```python
from build123d import *
from OCP.BRepFilletAPI import BRepFilletAPI_MakeChamfer

# Parameters (mm, degrees)
SKETCH1_W           = 46
SKETCH1_H           = 34
SKETCH1_R           = 4.5
BOSS_EXTRUDE1_DEPTH = 17
SKETCH2_W           = 45.8
SKETCH2_H           = 33.8
BOSS_EXTRUDE2_DEPTH = 2
SKETCH3_W           = 45.8
SKETCH3_H           = 33.8
BOSS_EXTRUDE3_DEPTH = 5
CHAMFER1_SIZE       = 5
CHAMFER1_SIZE2      = 4.346433689
SKETCH5_R           = 4.5
CUT_EXTRUDE1_DEPTH  = 63.032249677
CUT_EXTRUDE2_DEPTH  = 4
CUT_EXTRUDE3_DEPTH  = 4.5
CUT_EXTRUDE4_DEPTH  = 0.2
SKETCH11_W          = 11.4
SKETCH11_H          = 5
BOSS_EXTRUDE4_DEPTH = 4
SKETCH12_W          = 10.4
SKETCH12_H          = 1
CUT_EXTRUDE5_DEPTH  = 0.5
SKETCH13_W          = 10.4
SKETCH13_H          = 3
CUT_EXTRUDE6_DEPTH  = 0.5
SKETCH14_W          = 0.75
SKETCH14_H          = 2
BOSS_EXTRUDE5_DEPTH = 0.5
SKETCH15_W          = 0.75
SKETCH15_H          = 1
BOSS_EXTRUDE6_DEPTH = 1
SKETCH16_W          = 10.4
SKETCH16_H          = 3
BOSS_EXTRUDE7_DEPTH = 1
CUT_EXTRUDE7_DEPTH  = 1
SKETCH19_R          = 1
CUT_EXTRUDE8_DEPTH  = 2
SKETCH20_R          = 1.848835828
CUT_EXTRUDE9_DEPTH  = 2
BOSS_EXTRUDE8_DEPTH = 2
BOSS_EXTRUDE9_DEPTH = 2


with BuildPart() as part:
    # Sketch1 → Boss-Extrude1 (new body)
    with BuildSketch(Plane(origin=(0, 0, 0), x_dir=(1, 0, 0), z_dir=(0, 1, 0))):
        with Locations((23, 17)):
            Rectangle(SKETCH1_W, SKETCH1_H)
        with Locations(Location((23, 17, 0), (0, 0, 270))):
            Circle(SKETCH1_R, mode=Mode.SUBTRACT)
    extrude(amount=BOSS_EXTRUDE1_DEPTH)

    # Sketch2 → Boss-Extrude2 (add)
    with BuildSketch(Plane(origin=(0, 17, 0), x_dir=(1, 0, 0), z_dir=(0, 1, 0))):
        with Locations((23, 17)):
            Rectangle(SKETCH2_W, SKETCH2_H)
    extrude(amount=BOSS_EXTRUDE2_DEPTH)

    # Sketch3 → Boss-Extrude3 (add)
    with BuildSketch(Plane(origin=(0, 19, 0), x_dir=(1, 0, 0), z_dir=(0, 1, 0))):
        with Locations((23, 17)):
            Rectangle(SKETCH3_W, SKETCH3_H)
    extrude(amount=BOSS_EXTRUDE3_DEPTH)

    # Chamfer1: one chamfer whose edges measure the first distance from different faces: ONE call of the kernel's chamfer builder (chamfer() names one face for all edges)
    chamfer1_edges_1 = [part.edges().sort_by_distance(p)[0] for p in [
        (23, 24, -33.9),
    ]]
    chamfer1_side_1 = [part.faces().sort_by_distance(p)[0] for p in [
        (23, 20.5, -33.9),
    ]]
    chamfer1_edges_2 = [part.edges().sort_by_distance(p)[0] for p in [
        (0.1, 24, -17),
    ]]
    chamfer1_side_2 = [part.faces().sort_by_distance(p)[0] for p in [
        (0.1, 20.5, -17),
    ]]
    chamfer1_edges_3 = [part.edges().sort_by_distance(p)[0] for p in [
        (23, 24, -0.1),
    ]]
    chamfer1_side_3 = [part.faces().sort_by_distance(p)[0] for p in [
        (23, 20.5, -0.1),
    ]]
    chamfer1_edges_4 = [part.edges().sort_by_distance(p)[0] for p in [
        (45.9, 24, -17),
    ]]
    chamfer1_side_4 = [part.faces().sort_by_distance(p)[0] for p in [
        (45.9, 20.5, -17),
    ]]
    chamfer1 = BRepFilletAPI_MakeChamfer(part.part.solid().wrapped)
    for e in chamfer1_edges_1:
        chamfer1.Add(CHAMFER1_SIZE, CHAMFER1_SIZE2, e.wrapped, chamfer1_side_1[0].wrapped)  # the first distance lies on this face
    for e in chamfer1_edges_2:
        chamfer1.Add(CHAMFER1_SIZE, CHAMFER1_SIZE2, e.wrapped, chamfer1_side_2[0].wrapped)  # the first distance lies on this face
    for e in chamfer1_edges_3:
        chamfer1.Add(CHAMFER1_SIZE, CHAMFER1_SIZE2, e.wrapped, chamfer1_side_3[0].wrapped)  # the first distance lies on this face
    for e in chamfer1_edges_4:
        chamfer1.Add(CHAMFER1_SIZE, CHAMFER1_SIZE2, e.wrapped, chamfer1_side_4[0].wrapped)  # the first distance lies on this face
    add(Compound.cast(chamfer1.Shape()), mode=Mode.REPLACE)

    # Sketch5 → Cut-Extrude1 (cut, through all)
    with BuildSketch(Plane(origin=(0, 24, 0), x_dir=(1, 0, 0), z_dir=(0, 1, 0))):
        with Locations(Location((23, 17, 0), (0, 0, 270))):
            Circle(SKETCH5_R)
    extrude(amount=-CUT_EXTRUDE1_DEPTH, mode=Mode.SUBTRACT)

    # Sketch7 → Cut-Extrude2 (cut)
    with BuildSketch(Plane(origin=(0, 24, 0), x_dir=(1, 0, 0), z_dir=(0, 1, 0))):
        Polygon((41.375862069, 12.011652794), (41.553566311, 12.011652794), (41.553566311, 29.553566311), (22.9, 29.553566311), (27.975862069, 21.638287753), (27.975862069, 16.037336504), (41.375862069, 16.037336504), align=None)
        Polygon((45.9, 12.011652794), (45.9, 33.9), (22.9, 34), (22.9, 29.553566311), (41.553566311, 29.553566311), (41.553566311, 12.011652794), align=None)
    extrude(amount=-CUT_EXTRUDE2_DEPTH, mode=Mode.SUBTRACT)

    # Sketch9 → Cut-Extrude3 (cut)
    with BuildSketch(Plane(origin=(0, 24, 0), x_dir=(1, 0, 0), z_dir=(0, 1, 0))):
        with BuildLine():
            Line((0.1, 17), (0.1, 15.1))
            ThreePointArc((0.1, 15.1), (4.029878247, 13.643077531), (6.539387691, 17))
            Line((6.539387691, 17), (0.1, 17))
        make_face()
        with BuildLine():
            Line((0.1, 18.9), (0.1, 17))
            Line((0.1, 17), (6.539387691, 17))
            ThreePointArc((6.539387691, 17), (4.029878247, 20.356922469), (0.1, 18.9))
        make_face()
        with BuildLine():
            Line((0.1, 17), (0.1, 15.1))
            ThreePointArc((0.1, 15.1), (4.029878247, 13.643077531), (6.539387691, 17))
            Line((6.539387691, 17), (0.1, 17))
        make_face()
        with BuildLine():
            Line((0.1, 18.9), (0.1, 17))
            Line((0.1, 17), (6.539387691, 17))
            ThreePointArc((6.539387691, 17), (4.029878247, 20.356922469), (0.1, 18.9))
        make_face()
        with BuildLine():
            Line((0.1, 17), (0.1, 15.1))
            ThreePointArc((0.1, 15.1), (4.029878247, 13.643077531), (6.539387691, 17))
            Line((6.539387691, 17), (0.1, 17))
        make_face()
        with BuildLine():
            Line((0.1, 18.9), (0.1, 17))
            Line((0.1, 17), (6.539387691, 17))
            ThreePointArc((6.539387691, 17), (4.029878247, 20.356922469), (0.1, 18.9))
        make_face()
        with BuildLine():
            Line((0.1, 17), (0.1, 15.1))
            ThreePointArc((0.1, 15.1), (4.029878247, 13.643077531), (6.539387691, 17))
            Line((6.539387691, 17), (0.1, 17))
        make_face()
        with BuildLine():
            Line((0.1, 18.9), (0.1, 17))
            Line((0.1, 17), (6.539387691, 17))
            ThreePointArc((6.539387691, 17), (4.029878247, 20.356922469), (0.1, 18.9))
        make_face()
    extrude(amount=-CUT_EXTRUDE3_DEPTH, mode=Mode.SUBTRACT)

    # Sketch10 → Cut-Extrude4 (cut)
    with BuildSketch(Plane(origin=(0, 20, 0), x_dir=(1, 0, 0), z_dir=(0, 1, 0))):
        with BuildLine():
            Line((43.030713262, 22.3), (42.5, 22.3))
            ThreePointArc((42.5, 22.3), (41.792893219, 22.007106781), (41.5, 21.3))
            Line((41.5, 21.3), (41.5, 16.641494247))
            Line((41.5, 16.641494247), (28.1, 16.641494247))
            Line((28.1, 16.641494247), (28.1, 21.726215688))
            Line((28.1, 21.726215688), (22.9, 29.641494247))
            Line((22.9, 29.641494247), (22.9, 31.6))
            Line((22.9, 31.6), (43.030713262, 31.6))
            Line((43.030713262, 31.6), (43.030713262, 22.3))
        make_face()
    extrude(amount=-CUT_EXTRUDE4_DEPTH, mode=Mode.SUBTRACT)

    # Sketch11 → Boss-Extrude4 (add)
    with BuildSketch(Plane(origin=(0, 19.8, 0), x_dir=(1, 0, 0), z_dir=(0, 1, 0))):
        with Locations((34.8, 21.141494247)):
            Rectangle(SKETCH11_W, SKETCH11_H)
    extrude(amount=BOSS_EXTRUDE4_DEPTH)

    # Sketch12 → Cut-Extrude5 (cut)
    with BuildSketch(Plane(origin=(0, 23.8, 0), x_dir=(1, 0, 0), z_dir=(0, 1, 0))):
        with Locations((34.8, 19.141494247)):
            Rectangle(SKETCH12_W, SKETCH12_H)
    extrude(amount=-CUT_EXTRUDE5_DEPTH, mode=Mode.SUBTRACT)

    # Sketch13 → Cut-Extrude6 (cut)
    with BuildSketch(Plane.XY.offset(-18.641494247)):
        with Locations((34.8, 21.3)):
            Rectangle(SKETCH13_W, SKETCH13_H)
    extrude(amount=-CUT_EXTRUDE6_DEPTH, mode=Mode.SUBTRACT)

    # Sketch14 → Boss-Extrude5 (add)
    with BuildSketch(Plane.XY.offset(-19.141494247)):
        with Locations((30.475, 20.8)):
            Rectangle(SKETCH14_W, SKETCH14_H)
        with Locations((32.225, 20.8)):
            Rectangle(SKETCH14_W, SKETCH14_H)
        with Locations((33.975, 20.8)):
            Rectangle(SKETCH14_W, SKETCH14_H)
        with Locations((35.625, 20.8)):
            Rectangle(SKETCH14_W, SKETCH14_H)
        with Locations((37.375, 20.8)):
            Rectangle(SKETCH14_W, SKETCH14_H)
        with Locations((39.125, 20.8)):
            Rectangle(SKETCH14_W, SKETCH14_H)
    extrude(amount=BOSS_EXTRUDE5_DEPTH)

    # Sketch15 → Boss-Extrude6 (add)
    with BuildSketch(Plane.XY.offset(-18.641494247)):
        with Locations((30.475, 20.3)):
            Rectangle(SKETCH15_W, SKETCH15_H)
        with Locations((32.225, 20.3)):
            Rectangle(SKETCH15_W, SKETCH15_H)
        with Locations((33.975, 20.3)):
            Rectangle(SKETCH15_W, SKETCH15_H)
        with Locations((35.625, 20.3)):
            Rectangle(SKETCH15_W, SKETCH15_H)
        with Locations((37.375, 20.3)):
            Rectangle(SKETCH15_W, SKETCH15_H)
        with Locations((39.125, 20.3)):
            Rectangle(SKETCH15_W, SKETCH15_H)
    extrude(amount=BOSS_EXTRUDE6_DEPTH)

    # Sketch16 → Boss-Extrude7 (add)
    with BuildSketch(Plane(origin=(0, 0, -23.641494247), x_dir=(-1, 0, 0), z_dir=(0, 0, -1))):
        with Locations((-34.8, 21.8)):
            Rectangle(SKETCH16_W, SKETCH16_H)
    extrude(amount=BOSS_EXTRUDE7_DEPTH)

    # Sketch18 → Cut-Extrude7 (cut)
    with BuildSketch(Plane(origin=(0, 0, -24.641494247), x_dir=(-1, 0, 0), z_dir=(0, 0, -1))):
        Polygon((-38.5, 22.851547848), (-37.641246713, 22.851547848), (-37.641246713, 21.62271547), (-37.883028636, 21.62271547), (-37.883028636, 21.05), (-38.258218077, 21.05), (-38.258218077, 21.62271547), (-38.5, 21.62271547), align=None)
        Polygon((-35.782493426, 22.851547848), (-34.923740138, 22.851547848), (-34.923740138, 21.62271547), (-35.165522062, 21.62271547), (-35.165522062, 21.05), (-35.540711502, 21.05), (-35.540711502, 21.62271547), (-35.782493426, 21.62271547), align=None)
        Polygon((-37.141246713, 22.851547848), (-36.282493426, 22.851547848), (-36.282493426, 21.62271547), (-36.524275349, 21.62271547), (-36.524275349, 21.05), (-36.89946479, 21.05), (-36.89946479, 21.62271547), (-37.141246713, 21.62271547), align=None)
        Polygon((-34.423740138, 22.851547848), (-33.564986851, 22.851547848), (-33.564986851, 21.62271547), (-33.806768774, 21.62271547), (-33.806768774, 21.05), (-34.181958215, 21.05), (-34.181958215, 21.62271547), (-34.423740138, 21.62271547), align=None)
        Polygon((-33.064986851, 22.851547848), (-32.206233564, 22.851547848), (-32.206233564, 21.62271547), (-32.448015487, 21.62271547), (-32.448015487, 21.05), (-32.823204928, 21.05), (-32.823204928, 21.62271547), (-33.064986851, 21.62271547), align=None)
        Polygon((-31.706233564, 22.851547848), (-30.847480277, 22.851547848), (-30.847480277, 21.62271547), (-31.0892622, 21.62271547), (-31.0892622, 21.05), (-31.464451641, 21.05), (-31.464451641, 21.62271547), (-31.706233564, 21.62271547), align=None)
    extrude(amount=-CUT_EXTRUDE7_DEPTH, mode=Mode.SUBTRACT)

    # Sketch19 → Cut-Extrude8 (cut)
    with BuildSketch(Plane(origin=(0, 24, 0), x_dir=(1, 0, 0), z_dir=(0, 1, 0))):
        with Locations(Location((9.822889118, 16.294475275, 0), (0, 0, 270))):
            Circle(SKETCH19_R)
        with Locations(Location((12.479656801, 14.55031441, 0), (0, 0, 270))):
            Circle(SKETCH19_R)
        with Locations(Location((14.248903695, 12.19430902, 0), (0, 0, 270))):
            Circle(SKETCH19_R)
        with Locations(Location((15.225409883, 8.704826885, 0), (0, 0, 270))):
            Circle(SKETCH19_R)
        with Locations(Location((17.811892688, 6.813228664, 0), (0, 0, 270))):
            Circle(SKETCH19_R)
    extrude(amount=-CUT_EXTRUDE8_DEPTH, mode=Mode.SUBTRACT)

    # Sketch20 → Cut-Extrude9 (cut)
    with BuildSketch(Plane(origin=(0, 24, 0), x_dir=(1, 0, 0), z_dir=(0, 1, 0))):
        with Locations(Location((26.228756872, 7.901616706, 0), (0, 0, 270))):
            Circle(SKETCH20_R)
    extrude(amount=-CUT_EXTRUDE9_DEPTH, mode=Mode.SUBTRACT)

    # Sketch21 → Boss-Extrude8 (add)
    with BuildSketch(Plane.XZ):
        with BuildLine():
            Line((46, -34), (22.948134598, -34))
            Line((22.948134598, -34), (22.948134598, -35.5))
            ThreePointArc((22.948134598, -35.5), (23.094581208, -35.853553391), (23.448134598, -36))
            Line((23.448134598, -36), (45.5, -36))
            ThreePointArc((45.5, -36), (45.853553391, -35.853553391), (46, -35.5))
            Line((46, -35.5), (46, -34))
        make_face()
    extrude(amount=-BOSS_EXTRUDE8_DEPTH)

    # Sketch22 → Boss-Extrude9 (add)
    with BuildSketch(Plane.XZ):
        with BuildLine():
            Line((46, 0), (0, 0))
            Line((0, 0), (0, 1.328354237))
            ThreePointArc((0, 1.328354237), (0.196720489, 1.803279511), (0.671645763, 2))
            Line((0.671645763, 2), (45.328354237, 2))
            ThreePointArc((45.328354237, 2), (45.803279511, 1.803279511), (46, 1.328354237))
            Line((46, 1.328354237), (46, 0))
        make_face()
    extrude(amount=-BOSS_EXTRUDE9_DEPTH)


solid = part.part
```
Work out the finished part from the listing and answer in its coordinate system (mm). A direction names the side the tool comes from. Give positions to 0.01 mm unless a question says otherwise; leave off trailing zeros. Loops run counter-clockwise (first coordinate to the right, second up) from the corner with the lowest first, then second, coordinate; pieces in that order, holes last. Notation, with made-up numbers: (5, -4) -> (28, -4) arc R31 ccw to (28, 34) -> close; hole circle Ø8 at (23, 37). An arc over 180 degrees is marked (long way). Write item = value, one per line. Start each with the question number.
(1) Given pin 1 Ø10 at (x, y) = (30, 20) entering from -Z; pin 2 Ø1.1 at (y, z) = (22, -24) entering from +X; pin 3 Ø10 at (x, y) = (9.5, 15.5) entering from +Z, each flat-ended and moving along its own axis, determine where each tip first touches the part or whether it passes through.
(2) Find section B-B on z = -27. Give the vertices of the cut face in (x, y).
(3) Find section C-C on x = 6. Give the vertices of the cut face in (y, z).
(4) Find the intervals of material crossed by probe 1 along Z at (x, y) = (35.5, 16.5); probe 2 along Z at (x, y) = (35, 18); probe 3 along X at (y, z) = (23.25, -9), in increasing order. Write a range as from..to.
(5) The mould has two halves that part along Y. Classify faces 1 (the flat face through (18, 0, -17)), 2 (the flat face through (30.847, 22, -24)), 3 (the flat face through (35, 23.3, -19)): +Y half, -Y half, draft (parallel to the pull), parting line (faces both ways), or undercut.
(6) Find section A-A on y = 9. Give the vertices of the cut face in (x, z), and give its area (3 significant figures).
(7) Which of the six approach directions +Z, -Z, +X, -X, +Y, -Y give full straight-line access (tool end or side, diameter ignored) to faces 4 (the flat face through (34.35, 20.6, -18.6)), 5 (the flat face through (23, 18, -0.1)), 6 (the cylindrical face through (13.47, 23.01, -14.68)), 7 (the flat face through (45.9, 18, -17)), 8 (the flat face through (22.948, 1, -35))?
From the geometry:
q1.pin_1 = -34
q1.pin_2 = 40.5
q1.pin_3 = 0
q2.outline = (0, 0) -> (46, 0) -> (46, 17) -> (45.9, 17) -> (45.9, 19) -> (45.03, 20) -> (43.03, 20) -> (43.03, 19.8) -> (24.64, 19.8) -> (24.64, 20) -> (24.54, 20) -> (24.54, 24) -> (4.45, 24) -> (0.1, 19) -> (0.1, 17) -> (0, 17) -> close
q3.outline = (0, -34) -> (17, -34) -> (17, -33.9) -> (19, -33.9) -> (24, -29.55) -> (24, -18.87) -> (19.5, -18.87) -> (19.5, -15.13) -> (24, -15.13) -> (24, -4.45) -> (19, -0.1) -> (17, -0.1) -> (17, 0) -> (2, 0) -> (2, 2) -> (0, 2) -> close
q4.probe_1 = -34..0
q4.probe_2 = -33.9..-0.1
q4.probe_3 = 3.79..14.27, 16.18..24.74, 27.72..42.21
q5.face_1 = -Y half
q5.face_2 = undercut
q5.face_3 = +Y half
q6.outline = (0, -34) -> (46, -34) -> (46, 0) -> (0, 0) -> close; hole circle Ø9 at (23, -17)
q6.area = 1,500 mm^2
q7.face_4 = none
q7.face_5 = +Z, +X, -X, +Y
q7.face_6 = +Y
q7.face_7 = +Z, -Z, +X, +Y
q7.face_8 = -Z, -X, +Y, -Y
